Source: three-view drawing plus pictorial views. Frame: mm from the lowest corner of the part. A direction names the side the tool comes from. Round coordinates to 2 decimals unless told otherwise and drop trailing zeros. Loops run counter-clockwise (first coordinate to the right, second up) from the corner with the lowest first, then second, coordinate; pieces in that order, holes last. Notation, with made-up numbers: (12, 38.5) -> (20, 38.5) arc R15 cw to (20, 57.5) -> close; hole circle Ø4 at (-6.75, 2.25). An arc over 180 degrees is marked (long way). Answer in a Markdown table with one row per item. Add a question column.
Q1. Pin query (flat end, axial travel): pin 1 (17 mm diameter, centred on x = 124, y = 63.5, fed in from +Z). Return the tip coordinate at first contact, or that it passes through.
Q2. Ray query, L1, parallel to Y at x = 137, z = 150.5 (1 decimal); L2, parallel to X at y = 67, z = 145; L3, parallel to Z at x = 126, y = 62. Return the intervals inside material, ascending. Write a range as from..to.
Q3. Section C-C, the plane y = 45. Output: boundary loops of the cut face in (x, z) (1 decimal), and give its area (3 significant figures).
Q4. Mould query, pull axis Z, two halves, no side actions, for the marked faces 3, 4 and 5. Classes: pulls with the +Z half, pulls with the -Z half, needs draft (parallel to the pull), parting line crosses it, or undercut.
Q5. Section A-A, the plane y = 74. Output: boundary loops of the cut face in (x, z).
Q6. Section B-B, the plane x = 133.5. Output: boundary loops of the cut face in (y, z) (1 decimal).
Q7. Section D-D, the plane x = 51. Output: boundary loops of the cut face in (y, z) (1 decimal).
Q8. Reachability of the marked faces 1 and 2 from +Z, -Z, +X, -X, +Y, -Y: full face, straight path, thin tool, end or side. Return the list, or none.
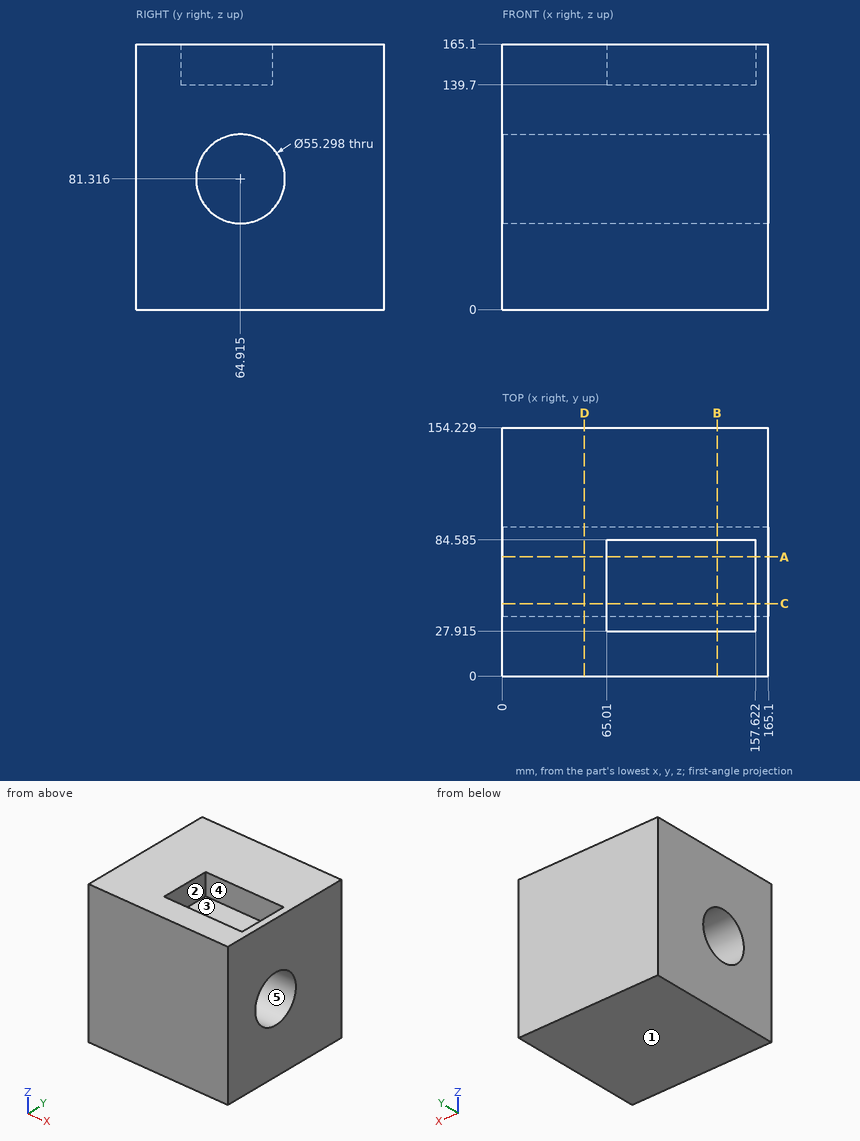
Answer block:
| question | item | result |
|---|---|---|
| 1 | pin 1 | z = 139.7 |
| 2 | L1 | 0..27.9, 84.6..154.2 |
| 2 | L2 | 0..65.01, 157.62..165.1 |
| 2 | L3 | 0..53.82, 108.81..139.7 |
| 3 | outline | (0, 0) -> (165.1, 0) -> (165.1, 62.1) -> (0, 62.1) -> close; (0, 100.5) -> (165.1, 100.5) -> (165.1, 165.1) -> (157.6, 165.1) -> (157.6, 139.7) -> (65, 139.7) -> (65, 165.1) -> (0, 165.1) -> close |
| 3 | area | 18,600 mm^2 |
| 4 | face 3 | pulls with the +Z half |
| 4 | face 4 | needs draft |
| 4 | face 5 | undercut |
| 5 | outline | (0, 0) -> (165.1, 0) -> (165.1, 55.2) -> (0, 55.2) -> close; (0, 107.43) -> (165.1, 107.43) -> (165.1, 165.1) -> (157.62, 165.1) -> (157.62, 139.7) -> (65.01, 139.7) -> (65.01, 165.1) -> (0, 165.1) -> close |
| 6 | outline | (0, 0) -> (154.2, 0) -> (154.2, 165.1) -> (84.6, 165.1) -> (84.6, 139.7) -> (27.9, 139.7) -> (27.9, 165.1) -> (0, 165.1) -> close; hole circle Ø55.3 at (64.9, 81.3) |
| 7 | outline | (0, 0) -> (154.2, 0) -> (154.2, 165.1) -> (0, 165.1) -> close; hole circle Ø55.3 at (64.9, 81.3) |
| 8 | face 1 | -Z, +X, -X, +Y, -Y |
| 8 | face 2 | +Z |
